Read the model definition and answer for the solid it produces. Units are mm, in the model's axes. A direction names the side the tool comes from. Coordinates: 2 decimals unless noted, no trailing zeros. Write each loop counter-clockwise with the first axis right and the second up, starting at its lowest first coordinate (ties: lowest second). Pieces come first, ordered by that corner, then holes. Notation, with made-up numbers: (-18.5, 12.5) - (-14.5, 12.5) arc R26 ccw to (-14.5, 32.5) - close; hole circle Ø6 at (3.25, 1). An arc over 180 degrees is marked (long way). Use a Markdown table: item, result.
from build123d import *

# Parameters (mm, degrees)
SKIZZE1_W                                            = 34
SKIZZE1_H                                            = 30
AUFSATZ_LINEAR_AUSTRAGEN1_DEPTH                      = 13
STIRNSENKUNG_F_R_M3_ZYLINDERSCHRAUBE_MIT_D           = 3.4
STIRNSENKUNG_F_R_M3_ZYLINDERSCHRAUBE_MIT_CBORE_D     = 6.5
STIRNSENKUNG_F_R_M3_ZYLINDERSCHRAUBE_MIT_CBORE_DEPTH = 3.4
SKIZZE4_W                                            = 8
SKIZZE4_H                                            = 27
AUFSATZ_LINEAR_AUSTRAGEN2_DEPTH                      = 30
F_4_0_4_DURCHMESSER_BOHRUNG1_AT_2_COUNT              = 2
F_4_0_4_DURCHMESSER_BOHRUNG1_AT_2_PITCH              = 17
SCHNITT_LINEAR_AUSTRAGEN1_DEPTH                      = 43
AUFSATZ_LINEAR_AUSTRAGEN3_DEPTH                      = 13
VERRUNDUNG2_R                                        = 3
VERRUNDUNG1_R                                        = 3
VERRUNDUNG4_R                                        = 1
F_4_0_4_DURCHMESSER_BOHRUNG2_D                       = 4
F_4_0_4_DURCHMESSER_BOHRUNG2_DEPTH                   = 5
F_4_0_4_DURCHMESSER_BOHRUNG2_TIP                     = 1.201721238


with BuildPart() as part:
    # Skizze1 → Aufsatz-Linear austragen1 (new body)
    with BuildSketch(Plane.XY):
        Rectangle(SKIZZE1_W, SKIZZE1_H)
    extrude(amount=AUFSATZ_LINEAR_AUSTRAGEN1_DEPTH)

    # Stirnsenkung für M3 Zylinderschraube mit Innensechskant1 (through all)
    with Locations(Plane.XY.offset(13)):
        with Locations((-12.5, 10), (-12.5, -10), (12.5, -10), (12.5, 10)):
            CounterBoreHole(STIRNSENKUNG_F_R_M3_ZYLINDERSCHRAUBE_MIT_D / 2, STIRNSENKUNG_F_R_M3_ZYLINDERSCHRAUBE_MIT_CBORE_D / 2, STIRNSENKUNG_F_R_M3_ZYLINDERSCHRAUBE_MIT_CBORE_DEPTH)

    # Skizze4 → Aufsatz-Linear austragen2 (add, through all)
    with BuildSketch(Plane(origin=(0, 15, 0), x_dir=(1, 0, 0), z_dir=(0, 1, 0))):
        with Locations((21, 0.5)):
            Rectangle(SKIZZE4_W, SKIZZE4_H)
    extrude(amount=-AUFSATZ_LINEAR_AUSTRAGEN2_DEPTH)

    # Skizze6 → Ø4.0 (4) Durchmesser Bohrung1 (revolve, cut)
    with BuildSketch(Plane(origin=(21, 15, 8), x_dir=(0, 0, 1), z_dir=(1, 0, 0))):
        Polygon((0, 0), (0, 6.201721238), (2, 5), (2, 0), align=None)
    f_4_0_4_durchmesser_bohrung1 = revolve(axis=Axis((21, 21.35, 8), (0, -1, 0)), mode=Mode.SUBTRACT)

    # Ø4.0 (4) Durchmesser Bohrung1 at 2: Ø4.0 (4) Durchmesser Bohrung1 ×2
    with Locations(*[(0, 0, -i * F_4_0_4_DURCHMESSER_BOHRUNG1_AT_2_PITCH) for i in range(1, F_4_0_4_DURCHMESSER_BOHRUNG1_AT_2_COUNT)]):
        add(f_4_0_4_durchmesser_bohrung1, mode=Mode.SUBTRACT)

    # Spiegeln1: Ø4.0 (4) Durchmesser Bohrung1 across plane
    add(f_4_0_4_durchmesser_bohrung1.mirror(Plane.ZX), mode=Mode.SUBTRACT)

    # Spiegeln1 copy 1 sketch → Spiegeln1 copy 1 (revolve, cut)
    with BuildSketch(Plane(origin=(21, -15, -9), x_dir=(0, 0, 1), z_dir=(1, 0, 0))):
        Polygon((0, 0), (0, -6.201721238), (2, -5), (2, 0), align=None)
    revolve(axis=Axis((21, -21.35, -9), (0, -1, 0)), mode=Mode.SUBTRACT)

    # Skizze7 → Schnitt-Linear austragen1 (cut, through all)
    with BuildSketch(Plane.ZY.offset(17)):
        Polygon((13, 2.65), (6.8, 5.15), (6.8, -5.15), (13, -2.65), align=None)
    extrude(amount=-SCHNITT_LINEAR_AUSTRAGEN1_DEPTH, mode=Mode.SUBTRACT)

    # Skizze10 → Aufsatz-Linear austragen3 (add)
    with BuildSketch(Plane(origin=(0, 0, 0), x_dir=(-1, 0, 0), z_dir=(0, 0, -1))):
        Polygon((-12.5, 15), (-8.5, 15), (-8.5, 21), (8.5, 21), (8.5, 15), (12.5, 15), (12.5, 25), (-12.5, 25), align=None)
    extrude(amount=-AUFSATZ_LINEAR_AUSTRAGEN3_DEPTH)

    # Verrundung2
    verrundung2_edges = [part.edges().sort_by_distance(p)[0] for p in [
        (-17, 15, 6.5),
        (-17, -15, 6.5),
        (-12.5, 25, 6.5),
        (12.5, 25, 6.5),
    ]]
    fillet(verrundung2_edges, radius=VERRUNDUNG2_R)

    # Verrundung1
    verrundung1_edges = [part.edges().sort_by_distance(p)[0] for p in [
        (17, 0, -14),
        (25, 0, -14),
    ]]
    fillet(verrundung1_edges, radius=VERRUNDUNG1_R)

    # Verrundung4
    verrundung4_edges = [part.edges().sort_by_distance(p)[0] for p in [
        (4, 2.65, 13),
        (4, -2.65, 13),
        (4, -5.15, 6.8),
        (4, 5.15, 6.8),
    ]]
    fillet(verrundung4_edges, radius=VERRUNDUNG4_R)

    # Ø4.0 (4) Durchmesser Bohrung2
    with Locations(Plane.XY.offset(6.8)):
        with Locations((21, 0)):
            Hole(F_4_0_4_DURCHMESSER_BOHRUNG2_D / 2, depth=F_4_0_4_DURCHMESSER_BOHRUNG2_DEPTH)
            with Locations((0, 0, -(F_4_0_4_DURCHMESSER_BOHRUNG2_DEPTH + F_4_0_4_DURCHMESSER_BOHRUNG2_TIP / 2))):  # 118° drill point
                Cone(0, F_4_0_4_DURCHMESSER_BOHRUNG2_D / 2, F_4_0_4_DURCHMESSER_BOHRUNG2_TIP, mode=Mode.SUBTRACT)


solid = part.part
(1) A cutting plane is placed at A-A, the plane x = -5. Write down the section's boundary in (y, z).
Report:
| item | result |
|---|---|
| outline | (-15, 0) - (15, 0) - (15, 13) - (4.13, 13) arc R1 ccw to (3.2, 11.63) - (4.6, 8.17) arc R1 cw to (3.67, 6.8) - (-3.67, 6.8) arc R1 cw to (-4.6, 8.17) - (-3.2, 11.63) arc R1 ccw to (-4.13, 13) - (-15, 13) - close; (21, 0) - (25, 0) - (25, 13) - (21, 13) - close |
(2) A cutting plane is placed at B-B, the plane z = 4. Write down the section's boundary in (x, y).
Report:
| item | result |
|---|---|
| outline | (-17, -12) arc R3 ccw to (-14, -15) - (25, -15) - (25, 15) - (12.5, 15) - (12.5, 22) arc R3 ccw to (9.5, 25) - (-9.5, 25) arc R3 ccw to (-12.5, 22) - (-12.5, 15) - (-14, 15) arc R3 ccw to (-17, 12) - close; hole circle Ø3.4 at (-12.5, -10); hole circle Ø3.4 at (-12.5, 10); hole (-8.5, 15) - (8.5, 15) - (8.5, 21) - (-8.5, 21) - close; hole circle Ø3.4 at (12.5, -10); hole circle Ø3.4 at (12.5, 10); hole circle Ø4 at (21, 0) |
(3) The mould has two halves that part along Z. Classify faces 5 (the cylindrical face through (10.105, 12.197, 11.324)), 6 (the cylindrical face through (19, 13, 8)), 7 (the cylindrical face through (4.294, 4.505, 7.252)), 8 (the cylindrical face through (24.1, -0.21, -13.14)): pulls with the +Z half, pulls with the -Z half, needs draft (parallel to the pull), parting line crosses it, or undercut.
Report:
| item | result |
|---|---|
| face 5 | needs draft |
| face 6 | undercut |
| face 7 | undercut |
| face 8 | pulls with the -Z half |
(4) Straight lines are drawn through the part: L1, parallel to X at y = -11.1, z = -9; L2, parallel to X at y = 9.5, z = 2.25; L3, parallel to X at y = -8, z = 11.5. For each, find the intervals that lie inside material, in ascending order.
Report:
| item | result |
|---|---|
| L1 | x = 17 to 19, 23 to 25 |
| L2 | x = -17 to -14.12, -10.88 to 10.88, 14.12 to 25 |
| L3 | x = -17 to -15.06, -9.94 to 9.94, 15.06 to 25 |
(5) A cutting plane is placed at C-C, the plane z = -6.25. Write down the section's boundary in (x, y).
Report:
| item | result |
|---|---|
| outline | (17, -15) - (25, -15) - (25, 15) - (17, 15) - close |
(6) Each of these flat-tipped pins is pushed along its axis until it touches: P1, Ø2.5, axis at x = 21, y = 0, coming from the +Z side; P2, Ø2, axis at y = 18, z = 3.5, coming from the +X side; P3, Ø12, axis at y = 12.5, z = -5, coming from the -X side; P4, Ø5, axis at x = 21, z = -9, coming from the +Y side. Where does it stop, or does it pass through?
Report:
| item | result |
|---|---|
| P1 | stops at z = 1.35 |
| P2 | stops at x = 12.5 |
| P3 | stops at x = -17 |
| P4 | stops at y = 15 |
(7) For faces 1 (the cylindrical face through (-14.895, 12.197, 11.324)), 2 (the flat face through (-12.5, 18, 6)), 3 (the flat face through (12.5, 19, 6)), 4 (the flat face through (-8.5, 18, 6)), determine the directions among +Z, -Z, +X, -X, +Y, -Y from which every point of the face is accessible in a straight line to the end or side of a thin tool.
Report:
| item | result |
|---|---|
| face 1 | +Z |
| face 2 | +Z, -Z, -X, +Y |
| face 3 | +Z, -Z, +X, +Y |
| face 4 | +Z, -Z |
